Autodesk Inventor part; units mm, degrees
ref_plane "YZ Plane" through (0, 0, 0) normal (1, 0, 0) x (0, 1, 0)
ref_plane "XZ Plane" through (0, 0, 0) normal (0, 1, 0) x (-1, 0, 0)
ref_plane "XY Plane" through (0, 0, 0) normal (0, 0, 1) x (1, 0, 0)
sketch "Sketch1" plane through (0, 0, 0) normal (0, 0, 1) x (1, 0, 0)
  line L0 (-200, 100) -> (200, 100)
  line L1 (200, 100) -> (200, -100)
  line L2 (200, -100) -> (-200, -100)
  line L3 (-200, -100) -> (-200, 100)
  line L4 (-200, 100) -> (200, -100) construction
  line L5 (200, 100) -> (-200, -100) construction
  point P0 (0, 0)
  point P1 (0, 0)
  point P2 (0, 0)
  dimension "d25" = 400
  dimension "d26" = 200
extrude "Plate1" add sketch "Sketch1" along normal blind 5
sketch "Sketch5" plane through (-195, -100, 0) normal (-1, 0, 0) x (0, -1, 0)
  line L0 (-200, 0) -> (0, 0)
  line L1 (0, 0) -> (0, 50)
  line L2 (0, 50) -> (-200, 50)
  line L3 (-200, 50) -> (-200, 0)
edge flange "Flange2" height 50 angle 90 thickness 5 bend radius 5 thickness toward (-1, 0, 0) relief round relief width 5 relief depth 2.5 corner gap 5 corner form 0 edges at (-200, 0, 5) (200, 0, 5) (0, 100, 5) (0, -100, 5) wall of the first edge with corners at (-195, 100, 0) (-195, -100, 0) (-195, -100, 50) (-195, 100, 50)
bend "Bend2"
corner "Corner2"
sketch "Sketch6" plane through (0, 0, 5) normal (0, 0, 1) x (1, 0, 0)
  circle A0 centre (-75, 0) radius 16
  circle A1 centre (75, 0) radius 16
  line L0 (0, 0) -> (0, 55.0725) construction
  circle A2 centre (33.5, 41.5) radius 5
  circle A3 centre (116.5, 41.5) radius 5
  circle A4 centre (116.5, -41.5) radius 5
  circle A5 centre (33.5, -41.5) radius 5
  line L1 (75, 0) -> (-75, 0)
  line L2 (75, 0) -> (75, -40.8866)
  circle A6 centre (-33.5, 41.5) radius 5
  circle A7 centre (-116.5, 41.5) radius 5
  circle A8 centre (-116.5, -41.5) radius 5
  circle A9 centre (-33.5, -41.5) radius 5
  point P0 (-75, -40.8866)
  dimension "d37" = 32
  dimension "d38" = 150
  dimension "d55" = 10
  dimension "d56" = 83
  dimension "d57" = 83
extrude "Cut1" cut sketch "Sketch6" against normal blind 5
sketch "Sketch7" plane through (-194.2929, 100, 10) normal (0, 1, 0) x (1, 0, 0)
  circle A0 centre (194.2929, -20) radius 6.5
  line L0 (5, 5) -> (383.5858, 5)
  line L1 (383.5858, 5) -> (384.2929, 5)
  line L2 (384.2929, 5) -> (383.5858, 5)
  line L3 (383.5858, 5) -> (5, 5)
  line L4 (5, 5) -> (4.2929, 5)
  line L5 (4.2929, 5) -> (5, 5)
  point P0 (194.2929, 10)
  dimension "d41" = 13
  dimension "d42" = 25
extrude "Extrusion2" cut sketch "Sketch7" against normal through all
pattern_linear "Rectangular Pattern1" count 3 spacing 160 along (-1, 0, 0) of "Extrusion2" first direction both ways yes
sketch "Sketch8" plane through (0, 0, 0) normal (1, 0, 0) x (0, 1, 0)
  line L0 (-94.2929, 50) -> (94.2929, 50)
  circle A0 centre (0, 30) radius 6.5
  line L1 (89.2929, 5) -> (-89.2929, 5)
  point P0 (0, 0)
  dimension "d48" = 13
  dimension "d49" = 25
extrude "Extrusion3" cut sketch "Sketch8" along normal through all both and the other way through all
pattern_linear "Rectangular Pattern2" count 3 spacing 70 along (0, 1, 0) of "Extrusion3" first direction both ways yes
sketch "Sketch9" plane through (0, 0, 0) normal (0, 0, 1) x (1, 0, 0)
  line L0 (-233.1694, -164.5287) -> (298.5547, -164.5287)
  line L1 (298.5547, -164.5287) -> (298.5547, 258.31)
  line L2 (298.5547, 258.31) -> (-233.1694, 258.31)
  line L3 (-233.1694, 258.31) -> (-233.1694, -164.5287)
  circle A0 centre (-75, 0) radius 16
  line L4 (-130, -55) -> (-20, -55)
  line L5 (-20, -55) -> (-20, 55)
  line L6 (-20, 55) -> (-130, 55)
  line L7 (-130, 55) -> (-130, -55)
  line L8 (-130, -55) -> (-20, 55) construction
  line L9 (-20, -55) -> (-130, 55) construction
  circle A1 centre (-75, 0) radius 40
  point P0 (0, 0)
  dimension "d58" = 110
  dimension "d59" = 110
  dimension "d60" = 80
extrude "Extrusion4" cut sketch "Sketch9" along normal through all both and the other way through all
fillet "Corner Round1" radius 6 4 edges at (-130, -55, 2.5) (-130, 55, 2.5) (-20, 55, 2.5) (-20, -55, 2.5)
equation "\"d25\" = Гриндер_проходная_ширина + 2 * Гриндер_размер_фланца"
equation "\"d26\" = Гриндер_высота"
equation "\"d38\" = Гриндер_Валы_между_центрами"
equation "\"d57\" = d56"
equation "\"d39\" = Thickness"
equation "\"d41\" = Гриндер_диам_отврс_корпуса"
equation "\"d42\" = Гриндер_отступ_отврс_корпуса"
equation "\"d48\" = Гриндер_диам_отврс_корпуса"
equation "\"d49\" = Гриндер_отступ_отврс_корпуса"
equation "\"d2\" = Thickness"
equation "\"d27\" = BendReliefWidth"
equation "\"d28\" = BendReliefDepth"
equation "\"d29\" = MinimumRemnant"
equation "\"d30\" = TransitionRadius"
equation "\"d33\" = BendRadius"
equation "\"d34\" = CornerReliefSize"
equation "\"d36\" = JacobiRadiusSize"
equation "\"BendReliefWidth\" = Thickness"
equation "\"BendReliefDepth\" = 0.5 * Thickness"
equation "\"TransitionRadius\" = BendRadius"
equation "\"JacobiRadiusSize\" = BendRadius"
equation "\"GapSize\" = Thickness"
equation "\"Гриндер_отступ_отврс_корпуса\" = 25"
equation "\"Гриндер_диам_отврс_корпуса\" = 13"
equation "\"Гриндер_проходная_ширина\" = 320"
equation "\"Гриндер_проходная_длина\" = 320"
equation "\"Гриндер_высота\" = 200"
equation "\"Гриндер_размер_фланца\" = 40"
equation "\"Гриндер_Валы_между_центрами\" = 150"
properties part number "NDM-VOS 162 harrow plate 5" material "Stainless Steel"
Model file for the job. Use its own axes, mm. Coordinates: 2 decimals unless noted, no trailing zeros. Write each loop counter-clockwise with the first axis right and the second up, starting at its lowest first coordinate (ties: lowest second). Pieces come first, ordered by that corner, then holes. Notation, with made-up numbers: (-36.75, -37.75) - (-17.75, -37.75) arc R17 ccw to (-17.75, -24.75) - close; hole circle Ø10 at (-2.75, 14.25). An arc over 180 degrees is marked (long way). Write each question's results on one line, items separated by ' | '. Start each with the question number.
1) Cut at B-B (y = 0). Write the cut outline in (x, z), then the cut area to 3 significant figures.
2) Cut at A-A (x = -33.5). Write the cut outline in (y, z), then the cut area to 3 significant figures.
3) Cut at D-D (y = 41.5). Write the cut outline in (x, z), then the cut area to 3 significant figures.
4) Probe line 1 along Y through (x, z) = (-33.5, 2.85); line 2 along X through (y, z) = (-1, 1.5); line 3 along Y through (x, z) = (-30.5, 3.9). List the from-to ranges inside material, lowest first. Write a range as from..to.
5) Mould opens along Y. For faces 1 (the face through (-128.289, -53.196, 2.535)), 2 (the face through (-36.847, -12.015, 2.465)), 3 (the face through (-128.289, 53.196, 2.465)) say: pulls with the +Y half, pulls with the -Y half, needs draft (parallel to the pull), parting line crosses it, or undercut.
6) Cut at C-C (x = -75). Write the cut outline in (y, z).
7) Flat gauge pin, fed straight in: P1, Ø6, axis at x = -116.5, y = 41.5, coming from the +Z side. Where does the tip first touch, or does it go through?
Returned:
1) outline: (-130, 0) - (-115, 0) - (-115, 5) - (-130, 5) - close; (-35, 0) - (-20, 0) - (-20, 5) - (-35, 5) - close | area: 150 mm^2
2) outline: (-55, 0) - (-46.5, 0) - (-46.5, 5) - (-55, 5) - close; (-36.5, 0) - (36.5, 0) - (36.5, 5) - (-36.5, 5) - close; (46.5, 0) - (55, 0) - (55, 5) - (46.5, 5) - close | area: 450 mm^2
3) outline: (-130, 0) - (-121.5, 0) - (-121.5, 5) - (-130, 5) - close; (-111.5, 0) - (-38.5, 0) - (-38.5, 5) - (-111.5, 5) - close; (-28.5, 0) - (-20, 0) - (-20, 5) - (-28.5, 5) - close | area: 450 mm^2
4) line 1: -55..-46.5, -36.5..36.5, 46.5..55 | line 2: -130..-114.99, -35.01..-20 | line 3: -55..-45.5, -37.5..37.5, 45.5..55
5) face 1: pulls with the -Y half | face 2: undercut | face 3: pulls with the +Y half
6) outline: (-55, 0) - (-40, 0) - (-40, 5) - (-55, 5) - close; (40, 0) - (55, 0) - (55, 5) - (40, 5) - close
7) P1: through
